```python
from build123d import *

# Parameters (mm, degrees)
BOSS_EXTRUDE1_DEPTH          = 48.41875
F_10_0_1935_DIAMETER_HOLE1_D = 4.9149
CUT_EXTRUDE3_REACH           = 65.246
SKETCH9_W                    = 63.5
SKETCH9_H                    = 6.35
CUT_EXTRUDE1_REACH           = 66.038
SKETCH7_W                    = 6.35
SKETCH7_H                    = 3.175
CUT_EXTRUDE2_REACH           = 65.246
SKETCH8_W                    = 6.35
SKETCH8_H                    = 3.175
FILLET1_R                    = 3.175
FILLET2_R                    = 3.175


with BuildPart() as part:
    # Sketch1 → Boss-Extrude1 (new, symmetric)
    with BuildSketch(Plane(origin=(0, 0, 0), x_dir=(0, 0, -1), z_dir=(1, 0, 0))):
        Polygon((0, 0), (-3.175, 0), (-3.175, 38.1), (14.2875, 38.1), (14.2875, 34.925), (0, 34.925), align=None)
    extrude(amount=BOSS_EXTRUDE1_DEPTH, both=True)

    # #10 (0.1935) Diameter Hole1 (through all)
    with Locations(Plane(origin=(0, 34.925, 0), x_dir=(-1, 0, 0), z_dir=(0, -1, 0))):
        with Locations((41.794904569, 7.239), (-42.06875, 6.35)):
            Hole(F_10_0_1935_DIAMETER_HOLE1_D / 2)

    # Sketch9 → Cut-Extrude3 (cut, up to next)
    with BuildSketch(Plane(origin=(0, 38.1, 0), x_dir=(1, 0, 0), z_dir=(0, 1, 0)), mode=Mode.PRIVATE) as cut_extrude3_sk1:
        with Locations((0, 11.1125)):
            Rectangle(SKETCH9_W, SKETCH9_H)
    cut_extrude3_tool1 = extrude(cut_extrude3_sk1.sketch, amount=-CUT_EXTRUDE3_REACH, mode=Mode.PRIVATE) & part.part
    add(cut_extrude3_tool1.solids().sort_by_distance((0, 38.1, -11.1125))[0], mode=Mode.SUBTRACT)

    # Sketch7 → Cut-Extrude1 (cut, up to next)
    with BuildSketch(Plane.XY.offset(3.175), mode=Mode.PRIVATE) as cut_extrude1_sk1:
        with Locations((-22.075650032, 1.5875)):
            Rectangle(SKETCH7_W, SKETCH7_H)
    cut_extrude1_tool1 = extrude(cut_extrude1_sk1.sketch, amount=-CUT_EXTRUDE1_REACH, mode=Mode.PRIVATE) & part.part
    # Sketch7 → Cut-Extrude1 (cut, up to next)
    with BuildSketch(Plane.XY.offset(3.175), mode=Mode.PRIVATE) as cut_extrude1_sk2:
        with Locations((22.075650032, 1.5875)):
            Rectangle(SKETCH7_W, SKETCH7_H)
    cut_extrude1_tool2 = extrude(cut_extrude1_sk2.sketch, amount=-CUT_EXTRUDE1_REACH, mode=Mode.PRIVATE) & part.part
    add(cut_extrude1_tool1.solids().sort_by_distance((-22.07565, 1.5875, 3.175))[0], mode=Mode.SUBTRACT)
    add(cut_extrude1_tool2.solids().sort_by_distance((22.07565, 1.5875, 3.175))[0], mode=Mode.SUBTRACT)

    # Sketch8 → Cut-Extrude2 (cut, up to next)
    with BuildSketch(Plane(origin=(0, 38.1, 0), x_dir=(1, 0, 0), z_dir=(0, 1, 0)), mode=Mode.PRIVATE) as cut_extrude2_sk1:
        with Locations((-22.071804601, 6.35)):
            Rectangle(SKETCH8_W, SKETCH8_H)
    cut_extrude2_tool1 = extrude(cut_extrude2_sk1.sketch, amount=-CUT_EXTRUDE2_REACH, mode=Mode.PRIVATE) & part.part
    # Sketch8 → Cut-Extrude2 (cut, up to next)
    with BuildSketch(Plane(origin=(0, 38.1, 0), x_dir=(1, 0, 0), z_dir=(0, 1, 0)), mode=Mode.PRIVATE) as cut_extrude2_sk2:
        with Locations((22.345650032, 6.35)):
            Rectangle(SKETCH8_W, SKETCH8_H)
    cut_extrude2_tool2 = extrude(cut_extrude2_sk2.sketch, amount=-CUT_EXTRUDE2_REACH, mode=Mode.PRIVATE) & part.part
    add(cut_extrude2_tool1.solids().sort_by_distance((-22.071805, 38.1, -6.35))[0], mode=Mode.SUBTRACT)
    add(cut_extrude2_tool2.solids().sort_by_distance((22.34565, 38.1, -6.35))[0], mode=Mode.SUBTRACT)

    # Fillet1
    fillet1_edges = [part.edges().sort_by_distance(p)[0] for p in [
        (25.250650032, 0, 1.5875),
        (18.900650032, 0, 1.5875),
        (-18.900650032, 0, 1.5875),
        (-25.250650032, 0, 1.5875),
        (48.41875, 36.5125, -14.2875),
        (-48.41875, 36.5125, -14.2875),
        (48.41875, 0, 1.5875),
        (-48.41875, 0, 1.5875),
        (25.520650032, 36.5125, -7.9375),
        (19.170650032, 36.5125, -7.9375),
        (-18.896804601, 36.5125, -7.9375),
        (-25.246804601, 36.5125, -7.9375),
        (31.75, 36.5125, -14.2875),
        (-31.75, 36.5125, -14.2875),
    ]]
    fillet(fillet1_edges, radius=FILLET1_R - 0.0001)  # a hair under: the kernel refuses the full size

    # Fillet2
    fillet2_edges = [part.edges().sort_by_distance(p)[0] for p in [
        (25.250650032, 3.175, 1.5875),
        (18.900650032, 3.175, 1.5875),
        (-18.900650032, 3.175, 1.5875),
        (-25.250650032, 3.175, 1.5875),
        (25.520650032, 36.5125, -4.7625),
        (19.170650032, 36.5125, -4.7625),
        (-18.896804601, 36.5125, -4.7625),
        (-25.246804601, 36.5125, -4.7625),
        (-31.75, 36.5125, -7.9375),
        (31.75, 36.5125, -7.9375),
    ]]
    fillet(fillet2_edges, radius=FILLET2_R)


solid = part.part
```
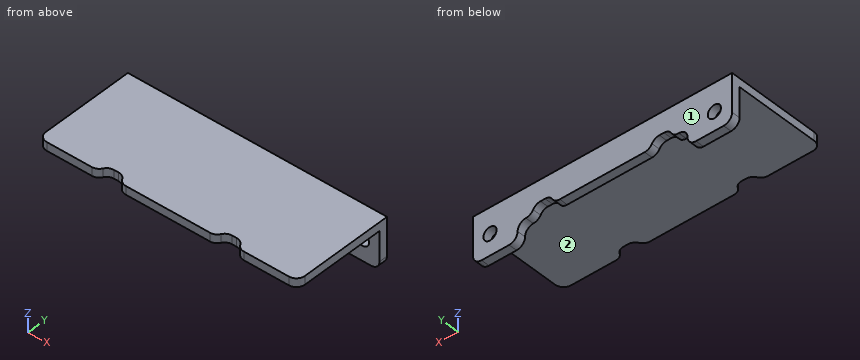
Verification items for the finished model (mm, model axes). Face numbers are marked on the shaded views. A direction names the side the tool comes from. Round coordinates to 2 decimals unless told otherwise and drop trailing zeros. Write each loop counter-clockwise with the first axis right and the second up, starting at its lowest first coordinate (ties: lowest second). Pieces come first, ordered by that corner, then holes. Notation, with made-up numbers: (72.5, 75) -> (108.5, 75) arc R30 ccw to (108.5, 107) -> close; hole circle Ø1 at (71, 59). An arc over 180 degrees is marked (long way). Write each question's results on one line, items separated by ' | '.
Q1. Go/stop test with flat-tipped pins: pin 1 Ø0.9 at (x, y) = (22.5, 36.5) entering from -Z; pin 2 Ø6.5 at (x, z) = (42.07, -6.35) entering from -Y (3 decimals); pin 3 Ø1.9 at (x, z) = (-22, 1.5) entering from -Y; pin 4 Ø10 at (y, z) = (12, -5.5) entering from +X. Record where each tip stops, or that it passes through.
Derived:
pin 1: stops at z = -4.76 | pin 2: stops at y = 34.925 | pin 3: stops at y = 3.17 | pin 4: passes through
Q2. Sectioned sample at A-A, the plane z = -13. Record the boundary of the cut face in (x, y) (3 decimals).
Derived:
outline: (-47.797, 34.925) -> (-32.372, 34.925) -> (-32.372, 38.1) -> (-47.797, 38.1) -> close; (32.372, 34.925) -> (47.797, 34.925) -> (47.797, 38.1) -> (32.372, 38.1) -> close
Q3. Thickness scan on probe 1 along Z at (x, y) = (27, 2) (3 decimals); probe 2 along Y at (x, z) = (-37, -1.25) (3 decimals); probe 3 along Z at (x, y) = (-9.5, 35.5) (1 decimal). Record the ranges inside material, lowest first.
Derived:
probe 1: z = 0 to 3.175 | probe 2: y = 34.925 to 38.1 | probe 3: z = -7.9 to 3.2
Q4. Sectioned sample at C-C, the plane y = 25. Record the boundary of the cut face in (x, z) (3 decimals), and give its area (3 significant figures).
Derived:
outline: (-48.419, 0) -> (48.419, 0) -> (48.419, 3.175) -> (-48.419, 3.175) -> close | area: 307 mm²
Q5. Sectioned sample at B-B, the plane x = 36. Record the boundary of the cut face in (y, z) (1 decimal), and give its area (3 significant figures).
Derived:
outline: (0, 0) -> (34.9, 0) -> (34.9, -14.3) -> (38.1, -14.3) -> (38.1, 3.2) -> (0, 3.2) -> close | area: 166 mm²
Q6. Access from +Z, -Z, +X, -X, +Y, -Y to the whole of each face (thin tool, end or side, straight path). Record for the marked faces 1 and 2.
Derived:
face 1: +Z, -Z, +X, -X, +Y | face 2: -Z, +X, -X, -Y
